The listing builds one solid part. Answer for the finished solid, in the listing's coordinates (mm). Face numbers are marked on the shaded views. A direction names the side the tool comes from. Give positions to 0.01 mm unless a question says otherwise; leave off trailing zeros. Loops run counter-clockwise (first coordinate to the right, second up) from the corner with the lowest first, then second, coordinate; pieces in that order, holes last. Notation, with made-up numbers: (64.25, -35.75) - (94.25, -35.75) arc R25 ccw to (94.25, -1.75) - close; hole circle Ø6 at (2.5, 88.25). An arc over 180 degrees is marked (long way). Write item = value, one per line. Start each with the question number.
1) Which of the six approach directions +Z, -Z, +X, -X, +Y, -Y give full straight-line access (tool end or side, diameter ignored) to the marked faces 1 and 2?
2) The part is cut by section C-C on z = 0. Write down the section's boundary in (x, y).
3) Flat-ended cylindrical pins translate along their axes: P1, Ø6, axis at x = 26.5, y = 29.5, coming from the +Z side; P2, Ø12, axis at y = -11, z = 0, coming from the -X side; P3, Ø6.5, axis at y = 0, z = 41.7, coming from the -X side; P4, Ø2, axis at x = 10, z = 32.5, coming from the +Y side. Find the tip coordinate at first contact, or state that the pin passes through.
4) Consider probe 1 along Z at (x, y) = (25, 0); probe 2 along Y at (x, z) = (24, 42); probe 3 along Z at (x, y) = (22.5, -2.5). Determine where each line is inside the solid, lowest interval first.
5) The part is cut by section D-D on y = 18. Write down the section's boundary in (x, z).
6) The part is cut by section A-A on y = 0. Write down the section's boundary in (x, z).
7) The mould has two halves that part along Z. Classify the marked faces 3, 4 and 5: +Z half, -Z half, draft (parallel to the pull), parting line (faces both ways), or undercut.
8) The part is cut by section B-B on x = 11. Write down the section's boundary in (y, z), plus the area to 3 significant figures.
from build123d import *

# Parameters (mm, degrees)
F1_DEPTH      = 25.4
F1_DEPTH_BACK = 25.4
F2_DEPTH      = 38.1
F2_DEPTH_BACK = 38.1
F3_R          = 3.534221
F4_DEPTH      = 46.301903


with BuildPart() as f1:
    # F0 (on Front) → F1 (new body, two sides)
    with BuildSketch(Plane.XZ) as f1_sk:
        with BuildLine():
            ThreePointArc((0, 21.039158), (21.039158, 0), (0, -21.039158))
            Line((0, -21.039158), (0, -30.469209))
            ThreePointArc((0, -30.469209), (30.469209, 0), (0, 30.469209))
            Line((0, 30.469209), (0, 21.039158))
        make_face()
        with BuildLine():
            ThreePointArc((0, 30.469209), (30.469209, 0), (0, -30.469209))
            Line((0, -30.469209), (0, -52.990768))
            Line((0, -52.990768), (46.300903, -52.990768))
            Line((46.300903, -52.990768), (46.300903, 0))
            Line((46.300903, 0), (46.300903, 52.990768))
            Line((46.300903, 52.990768), (0, 52.990768))
            Line((0, 52.990768), (0, 30.469209))
        make_face()
    extrude(amount=F1_DEPTH)
    extrude(f1_sk.sketch, amount=-F1_DEPTH_BACK)

    # F0 (on Front) → F2 (join, two sides)
    with BuildSketch(Plane.XZ) as f2_sk:
        with BuildLine():
            ThreePointArc((0, 21.039158), (21.039158, 0), (0, -21.039158))
            Line((0, -21.039158), (0, -30.469209))
            ThreePointArc((0, -30.469209), (30.469209, 0), (0, 30.469209))
            Line((0, 30.469209), (0, 21.039158))
        make_face()
    extrude(amount=F2_DEPTH)
    extrude(f2_sk.sketch, amount=-F2_DEPTH_BACK)

    # F3 (on Right) → F4 (cut, through all)
    with BuildSketch(Plane.YZ):
        with Locations((0, -41.703153)):
            Circle(F3_R)
        with Locations((0, 41.703153)):
            Circle(F3_R)
    extrude(amount=F4_DEPTH, mode=Mode.SUBTRACT)


solid = f1.part
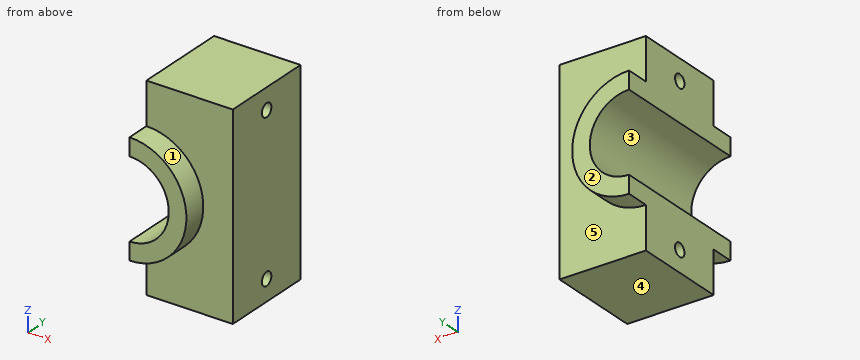
Answer below:
q1.face_1 = +X, -Y
q1.face_2 = +Z, -Z, +X, -X, +Y
q2.outline = (21.04, -38.1) - (30.47, -38.1) - (30.47, -25.4) - (46.3, -25.4) - (46.3, 25.4) - (30.47, 25.4) - (30.47, 38.1) - (21.04, 38.1) - close
q3.P1 = 19.39
q3.P2 = 20.17
q3.P3 = through
q3.P4 = 25.4
q4.probe_1 = -52.99 to -45.24, -38.17 to 38.17, 45.24 to 52.99
q4.probe_2 = -25.4 to -3.52, 3.52 to 25.4
q4.probe_3 = -52.99 to -44.2, -39.21 to 39.21, 44.2 to 52.99
q5.outline = (0, -52.99) - (46.3, -52.99) - (46.3, 52.99) - (0, 52.99) - (0, 21.04) arc R21.04 cw to (0, -21.04) - close
q6.outline = (0, -52.99) - (46.3, -52.99) - (46.3, -45.24) - (0, -45.24) - close; (0, -38.17) - (46.3, -38.17) - (46.3, 38.17) - (0, 38.17) - (0, 21.04) arc R21.04 cw to (0, -21.04) - close; (0, 45.24) - (46.3, 45.24) - (46.3, 52.99) - (0, 52.99) - close
q7.face_3 = undercut
q7.face_4 = -Z half
q7.face_5 = draft
q8.outline = (-38.1, -28.41) - (-25.4, -28.41) - (-25.4, -52.99) - (25.4, -52.99) - (25.4, -28.41) - (38.1, -28.41) - (38.1, -17.93) - (-38.1, -17.93) - close; (-38.1, 17.93) - (38.1, 17.93) - (38.1, 28.41) - (25.4, 28.41) - (25.4, 52.99) - (-25.4, 52.99) - (-25.4, 28.41) - (-38.1, 28.41) - close; hole circle Ø7.07 at (0, -41.7); hole circle Ø7.07 at (0, 41.7)
q8.area = 4,020 mm2
